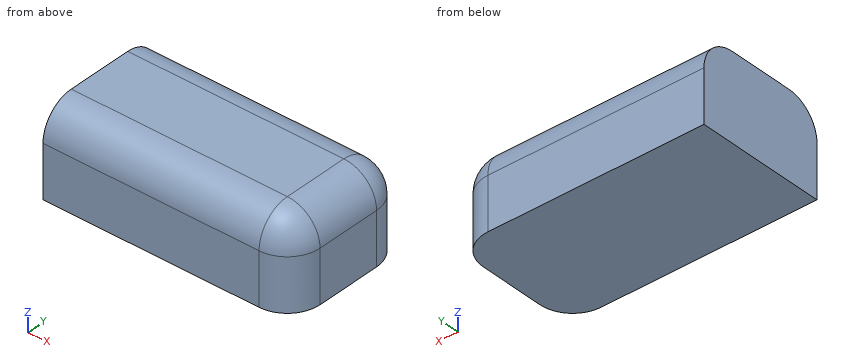
Autodesk Inventor part; units mm, degrees
ref_plane "YZ Plane" through (0, 0, 0) normal (1, 0, 0) x (0, 1, 0)
ref_plane "XZ Plane" through (0, 0, 0) normal (0, 1, 0) x (-1, 0, 0)
ref_plane "XY Plane" through (0, 0, 0) normal (0, 0, 1) x (1, 0, 0)
sketch "Sketch1" plane through (0, 0, 0) normal (1, 0, 0) x (0, 1, 0)
  line L0 (0, 0) -> (127, 0)
  line L1 (127, 0) -> (127, 50.8)
  line L2 (0, 0) -> (0, 50.8)
  arc A0 (95.25, 82.55) -> (127, 50.8) centre (95.25, 50.8) ccw construction
  arc A1 (31.75, 82.55) -> (0, 50.8) centre (31.75, 50.8) ccw
  line L3 (95.25, 82.55) -> (31.75, 82.55)
  arc A2 (127, 50.8) -> (95.25, 82.55) centre (95.25, 50.8) ccw
  line L4 (127, 19.05) -> (0, 19.05) construction
  dimension "d0" = 127
  dimension "d1" = 63.5
  dimension "d2" = 19.05
extrude "Extrusion1" add sketch "Sketch1" along normal blind 241.3
fillet "Fillet1" radius 31.75 5 edges at (241.3, 117.7006, 73.2506) (241.3, 63.5, 82.55) (241.3, 9.2994, 73.2506) (241.3, 0, 25.4) (241.3, 127, 25.4)
properties part number "Front Bumper"
The listing builds one solid part. Answer for the finished solid, in the listing's coordinates (mm). Coordinates: 2 decimals unless noted, no trailing zeros. Loops run counter-clockwise (first coordinate to the right, second up) from the corner with the lowest first, then second, coordinate; pieces in that order, holes last. Notation, with made-up numbers: M -20.5,37.5 L 37.5,37.5 A20 ccw 37.5,76.5 Z; hole C 69,25.5 d3. An arc over 180 degrees is marked long. Answer as a JSON object with one key per item and string values. Group by question number.
Item 1: Section A-A (x = 50) is taken. Write down the section's boundary in (y, z), and give its area (3 significant figures).
Item 2: Each of these flat-tipped pins is pushed along its axis until it touches: P1, Ø2, axis at y = 21, z = 25.5, coming from the +X side; P2, Ø4, axis at x = 69, y = 108, coming from the +Z side; P3, Ø10, axis at x = 86.5, z = 25.5, coming from the -Y side; P4, Ø1, axis at y = 87.5, z = 62.5, coming from the +X side. Where does it stop, or does it pass through?
Item 3: Section B-B (z = 70) is taken. Write down the section's boundary in (x, y).
Item 4: Consider L1, parallel to X at y = 15.5, z = 22; L2, parallel to Z at x = 127.5, y = 119.5; L3, parallel to X at y = 29.5, z = 45. Determine where each line is inside the solid, lowest interval first.
Item 5: Section C-C (y = 113.5) is taken. Write down the section's boundary in (x, z).
Solved:
{
 "1": {"outline": "M 0,0 L 127,0 L 127,50.8 A31.75 ccw 95.25,82.55 L 31.75,82.55 A31.75 ccw 0,50.8 Z", "area": "10,100 mm2"},
 "2": {"P1": "stops at x = 239.77", "P2": "stops at z = 80.67", "P3": "stops at y = 0", "P4": "stops at x = 239.26"},
 "3": {"outline": "M 0,6.46 L 209.55,6.46 A25.29 ccw 234.84,31.75 L 234.84,95.25 A25.29 ccw 209.55,120.54 L 0,120.54 Z"},
 "4": {"L1": "x = 0 to 236.83", "L2": "z = 0 to 71.29", "L3": "x = 0 to 241.22"},
 "5": {"outline": "M 0,0 L 235.53,0 L 235.53,50.8 A25.98 ccw 209.55,76.78 L 0,76.78 Z"}
}
